CAD build for the part. Positions are in the model's coordinates, mm. Give positions to 0.01 mm unless a question says otherwise; leave off trailing zeros.
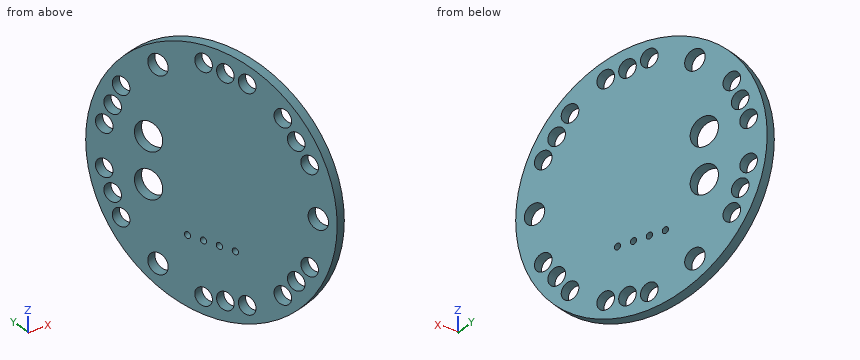
```python
from build123d import *

# Parameters (mm, degrees)
SKETCH1_R           = 20
BOSS_EXTRUDE1_DEPTH = 1.6
SKETCH2_R           = 1.625
CUT_EXTRUDE1_DEPTH  = 30.030785713
SKETCH3_R           = 1.4
CUT_EXTRUDE2_DEPTH  = 30.030785713
CIRPATTERN1_COUNT   = 3
SKETCH4_R           = 0.5
CUT_EXTRUDE3_DEPTH  = 30.030785713
SKETCH5_R           = 2.25
CUT_EXTRUDE4_DEPTH  = 30.030785713


with BuildPart() as part:
    # Sketch1 → Boss-Extrude1 (new body)
    with BuildSketch(Plane(origin=(-6.693944195, -2.366666667, 0), x_dir=(0, 0, -1), z_dir=(0.9428090415820737, 0.3333333333333042, 1.703606547556464e-15))):
        with Locations(Location((0, 0, 0), (0, 0, 90))):
            Circle(SKETCH1_R)
    extrude(amount=BOSS_EXTRUDE1_DEPTH)

    # Sketch2 → Cut-Extrude1 (cut, through all)
    with BuildSketch(Plane(origin=(-5.185449729, -1.833333333, 0), x_dir=(0, 0, -1), z_dir=(0.9428090415820737, 0.3333333333333043, 1.703606547556464e-15))):
        with Locations(Location((0, -17, 0), (0, 0, 90))):
            Circle(SKETCH2_R)
        with Locations(Location((-14.722431864, 8.5, 0), (0, 0, 90))):
            Circle(SKETCH2_R)
        with Locations(Location((14.722431864, 8.5, 0), (0, 0, 90))):
            Circle(SKETCH2_R)
    extrude(amount=-CUT_EXTRUDE1_DEPTH, mode=Mode.SUBTRACT)

    # Sketch3 → Cut-Extrude2 (cut, through all)
    with BuildSketch(Plane(origin=(-5.185449729, -1.833333333, 0), x_dir=(0, 0, -1), z_dir=(0.9428090415820736, 0.3333333333333042, 1.7036065475564638e-15))):
        with Locations(Location((-9.739196714, 14.366560039, 0), (0, 0, 90))):
            Circle(SKETCH3_R)
        with Locations(Location((-3.272039986, 17.045344066, 0), (0, 0, 90))):
            Circle(SKETCH3_R)
        with Locations(Location((-6.50561835, 15.705952053, 0), (0, 0, 90))):
            Circle(SKETCH3_R)
        with Locations(Location((9.739196714, 14.366560039, 0), (0, 0, 90))):
            Circle(SKETCH3_R)
        with Locations(Location((6.50561835, 15.705952053, 0), (0, 0, 90))):
            Circle(SKETCH3_R)
        with Locations(Location((3.272039986, 17.045344066, 0), (0, 0, 90))):
            Circle(SKETCH3_R)
    cut_extrude2 = extrude(amount=-CUT_EXTRUDE2_DEPTH, mode=Mode.SUBTRACT)

    # CirPattern1: Cut-Extrude2 ×3 about axis
    cirpattern1_axis = Axis((0, 0, 0), (0.9428090415820737, 0.3333333333333042, 1.703606547556464e-15))
    for i in range(1, CIRPATTERN1_COUNT):
        add(cut_extrude2.rotate(cirpattern1_axis, i * 360 / CIRPATTERN1_COUNT), mode=Mode.SUBTRACT)

    # Sketch4 → Cut-Extrude3 (cut, through all)
    with BuildSketch(Plane(origin=(-5.185449729, -1.833333333, 0), x_dir=(0, 0, -1), z_dir=(0.9428090415820736, 0.3333333333333042, 1.7036065475564638e-15))):
        with Locations(Location((9, 3.81, 0), (0, 0, 90))):
            Circle(SKETCH4_R)
        with Locations(Location((9, 1.27, 0), (0, 0, 90))):
            Circle(SKETCH4_R)
        with Locations(Location((9, -1.27, 0), (0, 0, 90))):
            Circle(SKETCH4_R)
        with Locations(Location((9, -3.81, 0), (0, 0, 90))):
            Circle(SKETCH4_R)
    extrude(amount=-CUT_EXTRUDE3_DEPTH, mode=Mode.SUBTRACT)

    # Sketch5 → Cut-Extrude4 (cut, through all)
    with BuildSketch(Plane(origin=(-5.185449729, -1.833333333, 0), x_dir=(0, 0, -1), z_dir=(0.9428090415820737, 0.3333333333333043, 1.703606547556464e-15))):
        with Locations(Location((-3.65, 10, 0), (0, 0, 90))):
            Circle(SKETCH5_R)
        with Locations(Location((3.45, 10, 0), (0, 0, 90))):
            Circle(SKETCH5_R)
    extrude(amount=-CUT_EXTRUDE4_DEPTH, mode=Mode.SUBTRACT)


solid = part.part
```
1. Drop flat-ended pins along their axis: pin 1 (2 mm diameter, centred on y = -0.5, z = -4.5, fed in from -X); pin 2 (12 mm diameter, centred on y = 12.5, z = -7, fed in from +X); pin 3 (6 mm diameter, centred on y = 0, z = 8.5, fed in from +X). Give the stop position or say it passes through.
Responses:
pin 1: stops at x = -7.71
pin 2: stops at x = -8.13
pin 3: stops at x = -4.77
2. Probe line 1 along X through (y, z) = (-8, 3); line 2 along X through (y, z) = (-3, -10); line 3 along Z through (x, y) = (-4, -9). List the from-to ranges inside material, lowest first.
Responses:
line 1: x = -4.7 to -3.01
line 2: x = -6.47 to -4.77
line 3: z = -18.68 to 18.68
3. Saw through at A-A, the plane y = 6. Count the separate pieces of the cut face and the enclosed holes in it, and give its area (3 significant figures).
Responses:
separate pieces: 5
enclosed holes: 0
area: 38.5 mm2
